from build123d import *

# Parameters (mm, degrees)
F0_W     = 20
F0_H     = 840
F1_DEPTH = 500
F3_DEPTH = 1397


with BuildPart() as f1:
    # F0 (on Front) → F1 (new body)
    with BuildSketch(Plane.XZ):
        with Locations((-2126.34038, 420)):
            Rectangle(F0_W, F0_H)
        Polygon((-2136.34038, 860), (-2136.34038, 840), (-2116.34038, 840), (398.65962, 840), (418.65962, 840), (418.65962, 860), align=None)
        with Locations((408.65962, 420)):
            Rectangle(F0_W, F0_H)
    extrude(amount=F1_DEPTH)

    # F2 (on Top) → F3 (cut)
    with BuildSketch(Plane.XY):
        with BuildLine():
            Line((-1621.34038, -470.847369), (-1051.34038, -470.847369))
            ThreePointArc((-1051.34038, -470.847369), (-1044.269312, -467.918437), (-1041.34038, -460.847369))
            Line((-1041.34038, -460.847369), (-1041.34038, -40.847369))
            ThreePointArc((-1041.34038, -40.847369), (-1044.269312, -33.776302), (-1051.34038, -30.847369))
            Line((-1051.34038, -30.847369), (-1621.34038, -30.847369))
            ThreePointArc((-1621.34038, -30.847369), (-1628.411448, -33.776302), (-1631.34038, -40.847369))
            Line((-1631.34038, -40.847369), (-1631.34038, -460.847369))
            ThreePointArc((-1631.34038, -460.847369), (-1628.411448, -467.918437), (-1621.34038, -470.847369))
        make_face()
    extrude(amount=F3_DEPTH, mode=Mode.SUBTRACT)


solid = f1.part
Source: CAD feature listing. Evaluate the final solid. Frame: model axes, mm. A direction names the side the tool comes from. Coordinates: 2 decimals unless noted, no trailing zeros. Order: outer loops, then holes, each group sorted by start corner. A loop starts at its lowest first (then second) coordinate and runs counter-clockwise, first axis right, second up.
Item 1: Cut plane B-B (z = 392). Return loops of the section in (x, y).
Output values:
outline: (-2136.34, -500) - (-2116.34, -500) - (-2116.34, 0) - (-2136.34, 0) - close; (398.66, -500) - (418.66, -500) - (418.66, 0) - (398.66, 0) - close
Item 2: Pull-direction query (X, two-part tool) for faces 3 (the face through (-2136.34, -246, 436)), 4 (the face through (398.66, -246, 414)), 5 (the face through (418.66, -246, 424)); classes: pulls with the +X half, pulls with the -X half, needs draft (parallel to the pull), parting line crosses it, or undercut.
Output values:
face 3: pulls with the -X half
face 4: undercut
face 5: pulls with the +X half
Item 3: Set-up query: faces 1 (the face through (-841, -246, 860)), 2 (the face through (-876, -246, 840)). Return all of +Z, -Z, +X, -X, +Y, -Y with unobstructed straight access to the full face (end or side cutting, diameter ignored); none if empty.
Output values:
face 1: +Z, +X, -X, +Y, -Y
face 2: -Z, +Y, -Y
Item 4: Material intervals for line 1 (X direction, y = -338.5, z = 161.5); line 2 (Z direction, x = -388.5, y = -225.5), sorted ascending.
Output values:
line 1: x = -2136.34 to -2116.34, 398.66 to 418.66
line 2: z = 840 to 860
Item 5: Cut plane A-A (y = -388). Return loops of the section in (x, z).
Output values:
outline: (-2136.34, 0) - (-2116.34, 0) - (-2116.34, 840) - (-1631.34, 840) - (-1631.34, 860) - (-2136.34, 860) - close; (-1041.34, 840) - (398.66, 840) - (398.66, 0) - (418.66, 0) - (418.66, 860) - (-1041.34, 860) - close
Item 6: Cut plane C-C (x = -715). Return loops of the section in (y, z), plus the area to 3 significant figures.
Output values:
outline: (-500, 840) - (0, 840) - (0, 860) - (-500, 860) - close
area: 10,000 mm2
